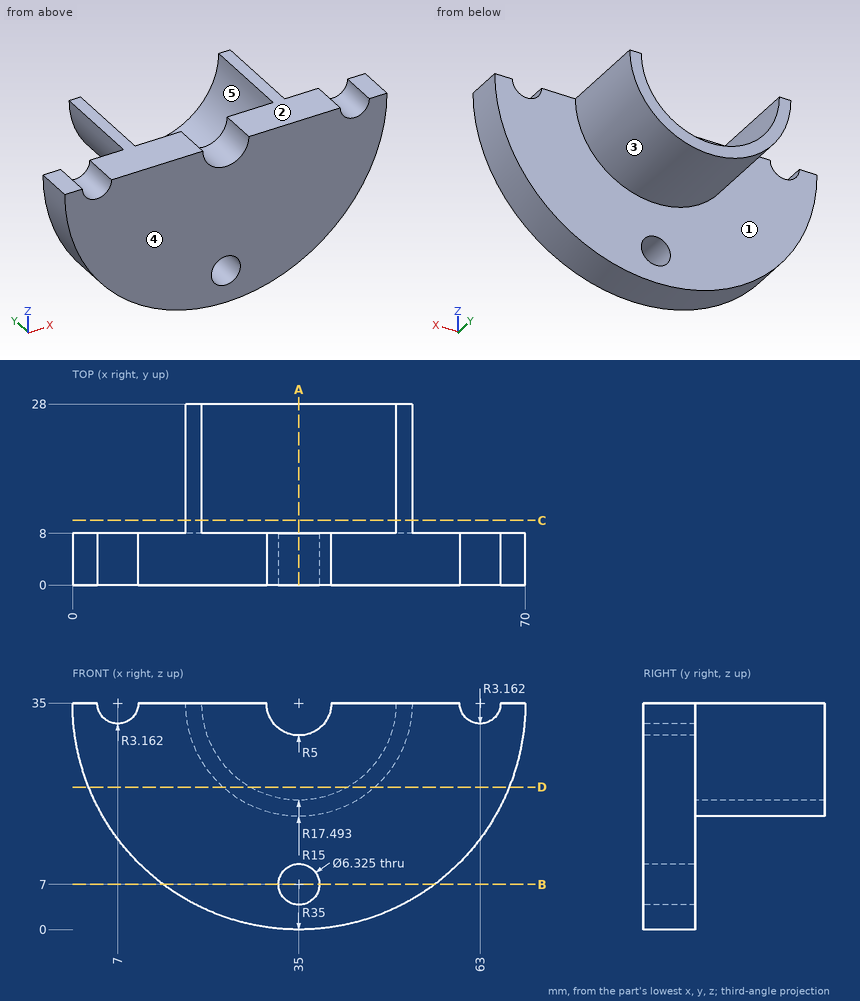
Source: three-view drawing plus pictorial views. Frame: mm from the lowest corner of the part. A direction names the side the tool comes from. Round coordinates to 2 decimals unless told otherwise and drop trailing zeros. Loops run counter-clockwise (first coordinate to the right, second up) from the corner with the lowest first, then second, coordinate; pieces in that order, holes last. Notation, with made-up numbers: M 10,66 L 53,66 A18 ccw 53,94 Z; hole C 49.25,87.25 d4. An arc over 180 degrees is marked long. Answer as CSV lines item,"result". Start each with the question number.
(1) First-contact query: pin 1 (1 mm diameter, centred on x = 15, y = 4.5, fed in from -Z) (1 decimal); pin 2 (10.5 mm diameter, centred on x = 46.5, z = 9.5, fed in from +Y); pin 3 (10 mm diameter, centred on y = 8, z = 21.5, fed in from +X). Flat tips, straight axial feed; report the tip coordinate or a pass-through.
(2) Draft query along X for the marked faces 3, 4 and 5. Return one class per face: released by +X, released by -X, zero draft, split by the parting line, or undercut.
(3) Reachability of the marked faces 1 and 2 from +Z, -Z, +X, -X, +Y, -Y: full face, straight path, thin tool, end or side. Return the list, or none.
(4) Section D-D, the plane z = 22. Output: boundary loops of the cut face in (x, y) (1 decimal).
(5) Section A-A, the plane x = 35. Output: boundary loops of the cut face in (y, z).
(6) Section B-B, the plane z = 7. Output: boundary loops of the cut face in (x, y), plus the area to 3 significant figures.
(7) Section C-C, the plane y = 10. Output: boundary loops of the cut face in (x, z) (1 decimal), plus the area to 3 significant figures.
(8) Line query: line 1 (X direction, y = 4.75, z = 33.5) (1 decimal); line 2 (Y direction, x = 60.5, z = 14); line 3 (X direction, y = 18, z = 26). Output: solid intervals per line, ascending. Write a range as [from, to].
Values found:
1,pin 1,"stops at z = 5.9"
1,pin 2,"stops at y = 8"
1,pin 3,"stops at x = 68.95"
2,face 3,"split by the parting line"
2,face 4,"zero draft"
2,face 5,"undercut"
3,face 1,"-Z, +Y"
3,face 2,"+Z, +X, -X, +Y, -Y"
4,outline,"M 2.5,0 L 67.5,0 L 67.5,8 L 46.7,8 L 46.7,28 L 42.5,28 L 42.5,8 L 27.5,8 L 27.5,28 L 23.3,28 L 23.3,8 L 2.5,8 Z"
5,outline,"M 0,0 L 8,0 L 8,3.84 L 0,3.84 Z; M 0,10.16 L 8,10.16 L 8,17.51 L 28,17.51 L 28,20 L 8,20 L 8,30 L 0,30 Z"
6,outline,"M 14,0 L 31.84,0 L 31.84,8 L 14,8 Z; M 38.16,0 L 56,0 L 56,8 L 38.16,8 Z"
6,area,"285 mm²"
7,outline,"M 17.5,35 A17.5 ccw 52.5,35 L 50,35 A15 cw 20,35 Z"
7,area,"127 mm²"
8,line 1,"x = [0, 4.2], [9.8, 30.2], [39.8, 60.2], [65.8, 70]"
8,line 2,"y = [0, 8]"
8,line 3,"x = [20, 23], [47, 50]"
